Build history of the part. All positions in model axes, mm. Face numbers are marked on the shaded views. A direction names the side the tool comes from. Round coordinates to 2 decimals unless told otherwise and drop trailing zeros. Loops run counter-clockwise (first coordinate to the right, second up) from the corner with the lowest first, then second, coordinate; pieces in that order, holes last. Notation, with made-up numbers: (16.5, -28.5) - (65.5, -28.5) arc R9 cw to (65.5, -12.5) - close; hole circle Ø2 at (-9, -16.5). An arc over 180 degrees is marked (long way). One line per question, with ' | ' between items. Start each with the question number.
Autodesk Inventor part; units mm, degrees
ref_plane "YZ Plane" through (0, 0, 0) normal (1, 0, 0) x (0, 1, 0)
ref_plane "XZ Plane" through (0, 0, 0) normal (0, 1, 0) x (-1, 0, 0)
ref_plane "XY Plane" through (0, 0, 0) normal (0, 0, 1) x (1, 0, 0)
sketch "Sketch1" plane through (0, 0, 0) normal (0, 1, 0) x (-1, 0, 0)
  line L0 (14.5, -14.5) -> (-14.5, -14.5)
  line L1 (-14.5, -14.5) -> (-14.5, 14.5)
  line L2 (-14.5, 14.5) -> (14.5, 14.5)
  line L3 (14.5, 14.5) -> (14.5, -14.5)
  dimension "d11" = 29
  dimension "d14" = 29
extrude "Extrusion1" add sketch "Sketch1" along normal blind 9
sketch "Sketch2" plane through (0, 9, 0) normal (0, 1, 0) x (1, 0, 0)
  line L0 (-5, 5) -> (5, 5)
  line L1 (5, 5) -> (5, -5)
  line L2 (5, -5) -> (-5, -5)
  line L3 (-5, -5) -> (-5, 5)
  line L4 (14.5, 14.5) -> (-14.5, 14.5)
  line L5 (14.5, -14.5) -> (14.5, 14.5)
  line L6 (-14.5, -14.5) -> (14.5, -14.5)
  line L7 (-14.5, 14.5) -> (-14.5, -14.5)
  point P0 (0, 0)
  dimension "d15" = 9.5
  dimension "d16" = 9.5
  dimension "d17" = 9.5
  dimension "d18" = 9.5
extrude "Extrusion2" add sketch "Sketch2" along normal blind 9 contours L0 L1 L2 L3
sketch "Sketch3" plane through (0, 0, 0) normal (0, -1, 0) x (1, 0, 0)
  line L0 (2.54, 1.778) -> (-2.54, 1.778)
  line L1 (-2.794, 1.524) -> (-2.794, -1.524)
  line L2 (-2.54, -1.778) -> (2.54, -1.778)
  line L3 (2.794, -1.524) -> (2.794, 1.524)
  arc A0 (2.794, 1.7526) -> (2.7686, 1.778) centre (2.7686, 1.7526) ccw
  arc A1 (2.794, 1.524) -> (2.54, 1.778) centre (2.54, 1.524) ccw
  arc A2 (2.54, -1.778) -> (2.794, -1.524) centre (2.54, -1.524) ccw
  arc A3 (-2.794, -1.524) -> (-2.54, -1.778) centre (-2.54, -1.524) ccw
  arc A4 (-2.54, 1.778) -> (-2.794, 1.524) centre (-2.54, 1.524) ccw
  point P0 (0, 0)
  point P1 (-0.254, 0)
  point P2 (-0.254, 0)
  dimension "d21" = 1.778
  dimension "d22" = 3.556
  dimension "d23" = 5.588
  dimension "d24" = 2.54
  dimension "d25" = 0.0254
  dimension "d26" = 0.254
  dimension "d27" = 2.794
  dimension "d28" = 1.778
extrude "Extrusion3" cut sketch "Sketch3" against normal blind 6
sketch "Sketch4" plane through (0, 0, 0) normal (0, -1, 0) x (1, 0, 0)
  point P0 (0, 0)
equation "\"d14\" = d11"
equation "\"d16\" = d15"
equation "\"d17\" = d15"
equation "\"d18\" = d15"
properties part number "Motor_fit_check"
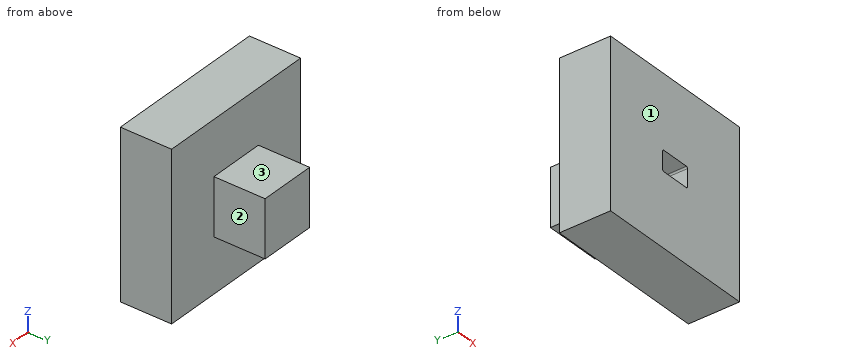
1) Saw through at A-A on y = 5.5. Write the cut outline in (x, z), and give its area (3 significant figures).
2) Tool access for the marked faces 1, 2 and 3: list every direction of +Z, -Z, +X, -X, +Y, -Y with a clear straight run to the whole face (end or side of a thin tool).
3) Wall check: line 1 (Z direction, x = 1, y = 2.25); line 2 (X direction, y = 0.5, z = 1); line 3 (Y direction, x = -4.75, z = 12). Give the ranges that are in metal, low to high. Write a range as [from, to].
4) Saw through at B-B on x = -0.75. Write the cut outline in (y, z), and give its area (3 significant figures).
5) Saw through at D-D on y = 10. Write the cut outline in (x, z), and give its area (3 significant figures).
6) Drop flat-ended pins along their axis: pin 1 (8 mm diameter, centred on y = 10, z = -10, fed in from -X); pin 2 (4.5 mm diameter, centred on y = 15.5, z = 0.5, fed in from +X); pin 3 (4.5 mm diameter, centred on y = 13.5, z = -0.5, fed in from -X); pin 4 (2.5 mm diameter, centred on x = -1.5, y = 12.5, fed in from +Z). Give the stop position or say it passes through.
7) Saw through at C-C on z = -2.25. Write the cut outline in (x, y), and give its area (3 significant figures).
Answer key:
1) outline: (-14.5, -14.5) - (14.5, -14.5) - (14.5, 14.5) - (-14.5, 14.5) - close; hole (-2.79, -1.52) arc R0.25 ccw to (-2.54, -1.78) - (2.54, -1.78) arc R0.25 ccw to (2.79, -1.52) - (2.79, 1.52) arc R0.25 ccw to (2.54, 1.78) - (-2.54, 1.78) arc R0.25 ccw to (-2.79, 1.52) - close | area: 821 mm²
2) face 1: +Z, -Z, +X, -X, -Y | face 2: +Z, -Z, +X, +Y | face 3: +Z, +X, -X, +Y
3) line 1: [-14.5, -1.78], [1.78, 14.5] | line 2: [-14.5, -2.79], [2.79, 14.5] | line 3: [0, 9]
4) outline: (0, -14.5) - (9, -14.5) - (9, -5) - (18, -5) - (18, 5) - (9, 5) - (9, 14.5) - (0, 14.5) - (0, 1.78) - (6, 1.78) - (6, -1.78) - (0, -1.78) - close | area: 330 mm²
5) outline: (-5, -5) - (5, -5) - (5, 5) - (-5, 5) - close | area: 100 mm²
6) pin 1: x = -14.5 | pin 2: x = 5 | pin 3: x = -5 | pin 4: z = 5
7) outline: (-14.5, 0) - (14.5, 0) - (14.5, 9) - (5, 9) - (5, 18) - (-5, 18) - (-5, 9) - (-14.5, 9) - close | area: 351 mm²
